```python
from build123d import *

# Parameters (mm, degrees)
F0_R     = 4.58
F1_DEPTH = 3


with BuildPart() as f1:
    # F0 (on Top) → F1 (new body)
    with BuildSketch(Plane.XY):
        with BuildLine():
            Line((14.711779, -2.926355), (33.094463, -2.926355))
            ThreePointArc((33.094463, -2.926355), (47.5, 0), (33.094463, 2.926355))
            Line((33.094463, 2.926355), (14.711779, 2.926355))
            Line((14.711779, 2.926355), (31.695164, 9.961103))
            ThreePointArc((31.695164, 9.961103), (43.884278, 18.177463), (29.455429, 15.368302))
            Line((29.455429, 15.368302), (12.472044, 8.333553))
            Line((12.472044, 8.333553), (25.470564, 21.332074))
            ThreePointArc((25.470564, 21.332074), (33.587572, 33.587572), (21.332074, 25.470564))
            Line((21.332074, 25.470564), (8.333553, 12.472044))
            Line((8.333553, 12.472044), (15.368302, 29.455429))
            ThreePointArc((15.368302, 29.455429), (18.177463, 43.884278), (9.961103, 31.695164))
            Line((9.961103, 31.695164), (2.926355, 14.711779))
            Line((2.926355, 14.711779), (2.926355, 33.094463))
            ThreePointArc((2.926355, 33.094463), (0, 47.5), (-2.926355, 33.094463))
            Line((-2.926355, 33.094463), (-2.926355, 14.711779))
            Line((-2.926355, 14.711779), (-9.961103, 31.695164))
            ThreePointArc((-9.961103, 31.695164), (-18.177463, 43.884278), (-15.368302, 29.455429))
            Line((-15.368302, 29.455429), (-8.333553, 12.472044))
            Line((-8.333553, 12.472044), (-21.332074, 25.470564))
            ThreePointArc((-21.332074, 25.470564), (-33.587572, 33.587572), (-25.470564, 21.332074))
            Line((-25.470564, 21.332074), (-12.472044, 8.333553))
            Line((-12.472044, 8.333553), (-29.455429, 15.368302))
            ThreePointArc((-29.455429, 15.368302), (-43.884278, 18.177463), (-31.695164, 9.961103))
            Line((-31.695164, 9.961103), (-14.711779, 2.926355))
            Line((-14.711779, 2.926355), (-33.094463, 2.926355))
            ThreePointArc((-33.094463, 2.926355), (-47.5, 0), (-33.094463, -2.926355))
            Line((-33.094463, -2.926355), (-14.711779, -2.926355))
            Line((-14.711779, -2.926355), (-31.695164, -9.961103))
            ThreePointArc((-31.695164, -9.961103), (-43.884278, -18.177463), (-29.455429, -15.368302))
            Line((-29.455429, -15.368302), (-12.472044, -8.333553))
            Line((-12.472044, -8.333553), (-25.470564, -21.332074))
            ThreePointArc((-25.470564, -21.332074), (-33.587572, -33.587572), (-21.332074, -25.470564))
            Line((-21.332074, -25.470564), (-8.333553, -12.472044))
            Line((-8.333553, -12.472044), (-15.368302, -29.455429))
            ThreePointArc((-15.368302, -29.455429), (-18.177463, -43.884278), (-9.961103, -31.695164))
            Line((-9.961103, -31.695164), (-2.926355, -14.711779))
            Line((-2.926355, -14.711779), (-2.926355, -33.094463))
            ThreePointArc((-2.926355, -33.094463), (0, -47.5), (2.926355, -33.094463))
            Line((2.926355, -33.094463), (2.926355, -14.711779))
            Line((2.926355, -14.711779), (9.961103, -31.695164))
            ThreePointArc((9.961103, -31.695164), (18.177463, -43.884278), (15.368302, -29.455429))
            Line((15.368302, -29.455429), (8.333553, -12.472044))
            Line((8.333553, -12.472044), (21.332074, -25.470564))
            ThreePointArc((21.332074, -25.470564), (33.587572, -33.587572), (25.470564, -21.332074))
            Line((25.470564, -21.332074), (12.472044, -8.333553))
            Line((12.472044, -8.333553), (29.455429, -15.368302))
            ThreePointArc((29.455429, -15.368302), (43.884278, -18.177463), (31.695164, -9.961103))
            Line((31.695164, -9.961103), (14.711779, -2.926355))
        make_face()
        with Locations((-28.284271, -28.284271)):
            Circle(F0_R, mode=Mode.SUBTRACT)
        with Locations((-15.307337, -36.955181)):
            Circle(F0_R, mode=Mode.SUBTRACT)
        with Locations((-36.955181, -15.307337)):
            Circle(F0_R, mode=Mode.SUBTRACT)
        with Locations((0, -40)):
            Circle(F0_R, mode=Mode.SUBTRACT)
        with Locations((15.307337, -36.955181)):
            Circle(F0_R, mode=Mode.SUBTRACT)
        with Locations((28.284271, -28.284271)):
            Circle(F0_R, mode=Mode.SUBTRACT)
        with Locations((36.955181, -15.307337)):
            Circle(F0_R, mode=Mode.SUBTRACT)
        with Locations((-40, 0)):
            Circle(F0_R, mode=Mode.SUBTRACT)
        with Locations((-36.955181, 15.307337)):
            Circle(F0_R, mode=Mode.SUBTRACT)
        with Locations((-28.284271, 28.284271)):
            Circle(F0_R, mode=Mode.SUBTRACT)
        with Locations((-15.307337, 36.955181)):
            Circle(F0_R, mode=Mode.SUBTRACT)
        with BuildLine():
            ThreePointArc((10.788638, 2.145994), (11, 0), (10.788638, -2.145994))
            ThreePointArc((10.788638, -2.145994), (10.162675, -4.209518), (9.146166, -6.111273))
            ThreePointArc((9.146166, -6.111273), (7.778175, -7.778175), (6.111273, -9.146166))
            ThreePointArc((6.111273, -9.146166), (4.209518, -10.162675), (2.145994, -10.788638))
            ThreePointArc((2.145994, -10.788638), (0, -11), (-2.145994, -10.788638))
            ThreePointArc((-2.145994, -10.788638), (-4.209518, -10.162675), (-6.111273, -9.146166))
            ThreePointArc((-6.111273, -9.146166), (-7.778175, -7.778175), (-9.146166, -6.111273))
            ThreePointArc((-9.146166, -6.111273), (-10.162675, -4.209518), (-10.788638, -2.145994))
            ThreePointArc((-10.788638, -2.145994), (-11, 0), (-10.788638, 2.145994))
            ThreePointArc((-10.788638, 2.145994), (-10.162675, 4.209518), (-9.146166, 6.111273))
            ThreePointArc((-9.146166, 6.111273), (-7.778175, 7.778175), (-6.111273, 9.146166))
            ThreePointArc((-6.111273, 9.146166), (-4.209518, 10.162675), (-2.145994, 10.788638))
            ThreePointArc((-2.145994, 10.788638), (0, 11), (2.145994, 10.788638))
            ThreePointArc((2.145994, 10.788638), (4.209518, 10.162675), (6.111273, 9.146166))
            ThreePointArc((6.111273, 9.146166), (7.778175, 7.778175), (9.146166, 6.111273))
            ThreePointArc((9.146166, 6.111273), (10.162675, 4.209518), (10.788638, 2.145994))
        make_face(mode=Mode.SUBTRACT)
        with Locations((40, 0)):
            Circle(F0_R, mode=Mode.SUBTRACT)
        with Locations((36.955181, 15.307337)):
            Circle(F0_R, mode=Mode.SUBTRACT)
        with Locations((0, 40)):
            Circle(F0_R, mode=Mode.SUBTRACT)
        with Locations((15.307337, 36.955181)):
            Circle(F0_R, mode=Mode.SUBTRACT)
        with Locations((28.284271, 28.284271)):
            Circle(F0_R, mode=Mode.SUBTRACT)
    extrude(amount=F1_DEPTH)


solid = f1.part
```
Source: CAD feature listing. Evaluate the final solid. Frame: model axes, mm. Coordinates: 2 decimals unless noted, no trailing zeros. Loops run counter-clockwise (first coordinate to the right, second up) from the corner with the lowest first, then second, coordinate; pieces in that order, holes last. Notation, with made-up numbers: (7, 23.25) - (58, 23.25) arc R17 ccw to (58, 43.25) - close; hole circle Ø3 at (23.25, 53). An arc over 180 degrees is marked (long way). Answer as CSV lines item,"result".
1. Section A-A (x = 0). Return loops of the section in (y, z).
Established:
outline,"(-47.5, 0) - (-44.58, 0) - (-44.58, 3) - (-47.5, 3) - close; (-35.42, 0) - (-11, 0) - (-11, 3) - (-35.42, 3) - close; (11, 0) - (35.42, 0) - (35.42, 3) - (11, 3) - close; (44.58, 0) - (47.5, 0) - (47.5, 3) - (44.58, 3) - close"
2. Contact query for flat-ended pins moving along their axis: pin 1 (1.5 mm diameter, centred on x = -4, z = 0.5, fed in from +Y); pin 2 (0.9 mm diameter, centred on y = 25.5, z = 1.5, fed in from -X); pin 3 (0.9 mm diameter, centred on y = -24.5, z = 2, fed in from +X). Output: stop coordinate, or through.
Established:
pin 1,"stops at y = 46.76"
pin 2,"stops at x = -35.41"
pin 3,"stops at x = 35"
3. Section C-C (x = -40). Return loops of the section in (y, z), then the cut area to 3 significant figures.
Established:
outline,"(-22.16, 0) - (-18.73, 0) - (-18.73, 3) - (-22.16, 3) - close; (-11.89, 0) - (-8.45, 0) - (-8.45, 3) - (-11.89, 3) - close; (-7.5, 0) - (-4.58, 0) - (-4.58, 3) - (-7.5, 3) - close; (4.58, 0) - (7.5, 0) - (7.5, 3) - (4.58, 3) - close; (8.45, 0) - (11.89, 0) - (11.89, 3) - (8.45, 3) - close; (18.73, 0) - (22.16, 0) - (22.16, 3) - (18.73, 3) - close"
area,"58.7 mm2"
4. Section B-B (y = 38.5). Return loops of the section in (x, z).
Established:
outline,"(-22.65, 0) - (-19.62, 0) - (-19.62, 3) - (-22.65, 3) - close; (-11, 0) - (-7.97, 0) - (-7.97, 3) - (-11, 3) - close; (-7.35, 0) - (-4.33, 0) - (-4.33, 3) - (-7.35, 3) - close; (4.33, 0) - (7.35, 0) - (7.35, 3) - (4.33, 3) - close; (7.97, 0) - (11, 0) - (11, 3) - (7.97, 3) - close; (19.62, 0) - (22.65, 0) - (22.65, 3) - (19.62, 3) - close"
5. Ray query, line 1 (Y direction, x = 36, z = 1.9); line 2 (Y direction, x = 43, z = 1.95); line 3 (X direction, y = -9.5, z = 0.7). Return the intervals inside material, ascending.
Established:
line 1,"y = -22.75 to -19.79, -10.83 to -7.87, -6.34 to -2.23, 2.23 to 6.34, 7.87 to 10.83, 19.79 to 22.75"
line 2,"y = -19.75 to -10.87, -6.87 to -3.46, 3.46 to 6.87, 10.87 to 19.75"
line 3,"x = -41.7 to -32.21, -30.58 to -15.29, -13.64 to -5.55, 5.55 to 13.64, 15.29 to 30.58, 32.21 to 41.7"
